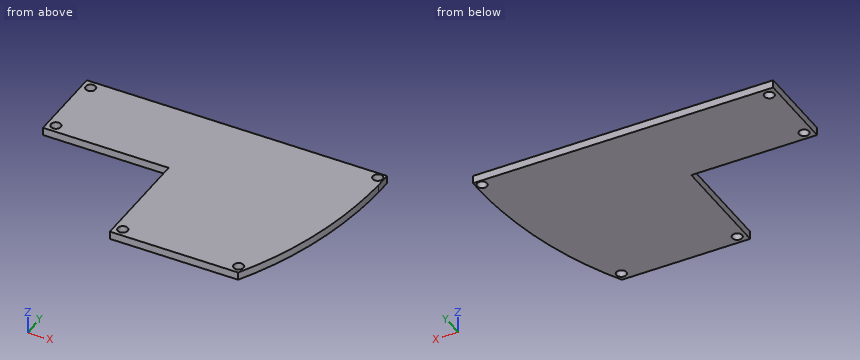
```python
from build123d import *

# Parameters (mm, degrees)
SKETCH_1_R      = 1
EXTRUDE_1_DEPTH = 1.6


with BuildPart() as part:
    # 草图1 → 凸台-拉伸1 (new body)
    with BuildSketch(Plane.XY):
        with BuildLine():
            Line((-87.7, -15.7), (-62.2, -15.7))
            Line((-62.2, -15.7), (-62.2, -37.7))
            Line((-62.2, -37.7), (-36.171688324, -37.7))
            add(Edge.make_bspline(
                [(-36.171688324, -37.7), (-34.684824725, -35.010251168), (-33.36902465, -32.239648029), (-31.086941159, -26.53324039), (-30.129135695, -23.618286004), (-28.96165245, -19.160150204), (-28.618715853, -17.664940446), (-28.023260614, -14.664637138), (-27.770339575, -13.158305121), (-27.140235066, -8.621562635), (-26.891543642, -5.573428708), (-26.8, -2.503618714)],
                knots=[0, 0, 0, 0, 0.25, 0.25, 0.5, 0.5, 0.625, 0.625, 0.75, 0.75, 1, 1, 1, 1], degree=3))
            Line((-26.8, -2.503618714), (-26.8, 0.7))
            Line((-26.8, 0.7), (-87.7, 0.7))
            Line((-87.7, 0.7), (-87.7, -15.7))
        make_face()
        with Locations((-86, -1)):
            Circle(SKETCH_1_R, mode=Mode.SUBTRACT)
        with Locations((-86, -14)):
            Circle(SKETCH_1_R, mode=Mode.SUBTRACT)
        with Locations((-28.008087081, -0.508087081)):
            Circle(SKETCH_1_R, mode=Mode.SUBTRACT)
        with Locations((-36.994977349, -36)):
            Circle(SKETCH_1_R, mode=Mode.SUBTRACT)
        with Locations((-60.5, -36)):
            Circle(SKETCH_1_R, mode=Mode.SUBTRACT)
    extrude(amount=EXTRUDE_1_DEPTH)


solid = part.part
```
Geometry check sheet. Reference: the model listing, model coordinates, mm. Give positions to 0.01 mm unless a question says otherwise; leave off trailing zeros. Order: outer loops, then holes, each group sorted by start corner. A loop starts at its lowest first (then second) coordinate and runs counter-clockwise, first axis right, second up. Notation, with made-up numbers: (41, 60) - (67, 60) arc R21 ccw to (67, 84) - close; hole circle Ø2 at (-6.75, 30). An arc over 180 degrees is marked (long way). Answer in a Markdown table with one row per item. Add a question column.
Q1. Material ranges on probe 1 along Y at (x, z) = (-86, 1.15); probe 2 along X at (y, z) = (-6.5, 0.5); probe 3 along Y at (x, z) = (-80, 1.35), recorded low to high. Write a range as from..to.
Q2. Cross-section at C-C, the plane y = -36. Count the separate pieces of the cut face and the enclosed holes in it, then the cut area to 3 significant figures.
Q3. Cross-section at A-A, the plane x = -86. Enter the section's corners in (y, z), then the cut area to 3 significant figures.
Q4. Cross-section at B-B, the plane x = -60.5. Enter the section's corners in (y, z), then the cut area to 3 significant figures.
Q5. Gauge pin test, flat ends, axial feed: pin 1 (0.8 mm diameter, centred on y = -31, z = 1, fed in from -X); pin 2 (0.5 mm diameter, centred on x = -71, z = 1, fed in from -Y). Record the tip position at first contact, or that the pin passes through.
Check values:
| question | item | result |
|---|---|---|
| 1 | probe 1 | y = -15.7..-15, -13..-2, 0..0.7 |
| 1 | probe 2 | x = -87.7..-27.01 |
| 1 | probe 3 | y = -15.7..0.7 |
| 2 | separate pieces | 3 |
| 2 | enclosed holes | 0 |
| 2 | area | 36.7 mm^2 |
| 3 | outline | (-15.7, 0) - (-15, 0) - (-15, 1.6) - (-15.7, 1.6) - close; (-13, 0) - (-2, 0) - (-2, 1.6) - (-13, 1.6) - close; (0, 0) - (0.7, 0) - (0.7, 1.6) - (0, 1.6) - close |
| 3 | area | 19.8 mm^2 |
| 4 | outline | (-37.7, 0) - (-37, 0) - (-37, 1.6) - (-37.7, 1.6) - close; (-35, 0) - (0.7, 0) - (0.7, 1.6) - (-35, 1.6) - close |
| 4 | area | 58.2 mm^2 |
| 5 | pin 1 | stops at x = -62.2 |
| 5 | pin 2 | stops at y = -15.7 |
